Read the model definition and answer for the solid it produces. Units are mm, in the model's axes. Face numbers are marked on the shaded views. A direction names the side the tool comes from. Give positions to 0.01 mm unless a question says otherwise; leave off trailing zeros. Loops run counter-clockwise (first coordinate to the right, second up) from the corner with the lowest first, then second, coordinate; pieces in that order, holes last. Notation, with made-up numbers: (82.5, 30) - (131.5, 30) arc R26 cw to (131.5, 51) - close; hole circle Ø8 at (4, 87.5). An arc over 180 degrees is marked (long way). Write each question's results on one line, items separated by ' | '. Start each with the question number.
Q1. Find the intervals of material crossed by line 1 (Y direction, x = 5, z = -6); line 2 (Y direction, x = -2, z = -7.5); line 3 (Z direction, x = -7.5, y = -39), in increasing order. Write a range as from..to.
Q2. Determine the mould class of the marked faces 1, 2 and 3 for opening direction X: +X half, -X half, draft (parallel to the pull), parting line (faces both ways), or undercut.
Q3. Given pin 1 (10 mm diameter, centred on y = -39.5, z = -2.5, fed in from +X); pin 2 (12 mm diameter, centred on x = -7.5, z = 21.5, fed in from +Y); pin 3 (13.5 mm diameter, centred on x = -7, y = -42.5, fed in from -Z); pin 4 (7.5 mm diameter, centred on x = 2.86, y = 9.6, fed in from +Z), each flat-ended and moving along its own axis, determine where each tip first touches the part or whether it passes through.
Q4. The part is cut by section B-B, the plane y = -26.5. Write down the section's boundary in (x, z) (3 decimals), plus the area to 3 significant figures.
Q5. For the marked faces 4, 5 and 6, determine the directions among +Z, -Z, +X, -X, +Y, -Y from which every point of the face is accessible in a straight line to the end or side of a thin tool.
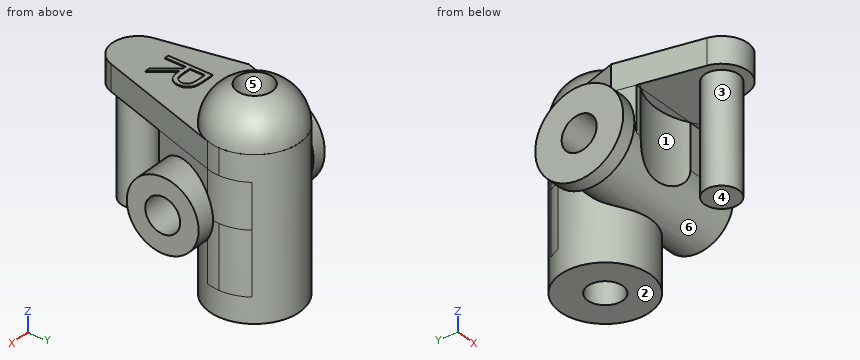
```python
from build123d import *
from build123d.topology import SkipClean

# Parameters (mm, degrees)
BOSS_EXTRU_1_DEPTH      = 1.45
ESQUISSE2_R             = 2.5
BOSS_EXTRU_2_DEPTH      = 2.2
BOSS_EXTRU_3_START      = -11.05
ESQUISSE3_R             = 2.5
BOSS_EXTRU_3_DEPTH      = 11.05
BOSS_EXTRU_4_START      = -1.45
ESQUISSE4_R             = 0.95
BOSS_EXTRU_4_DEPTH      = 7.5
CONG_1_R                = 2.2
BOSS_EXTRU_5_DEPTH      = 1
BOSS_EXTRU_5_DEPTH_BACK = 7.454
ENL_V_START             = -6
ENL_V_MAT_EXTRU_2_DEPTH = 6
BOSS_EXTRU_6_DEPTH      = 1
BOSS_EXTRU_6_DEPTH_BACK = 7.45
ESQUISSE8_R             = 2
ESQUISSE9_R             = 2.45
BOSS_EXTRU_7_DEPTH      = 0.8
ENL_V_START_2           = -6.05
ESQUISSE10_R            = 3.6
ESQUISSE10_R_2          = 0.95
ENL_V_MAT_EXTRU_3_DEPTH = 6.05
ESQUISSE11_R            = 0.975
ENL_V_MAT_EXTRU_4_DEPTH = 14.8
ESQUISSE12_R            = 0.975
ENL_V_MAT_EXTRU_5_DEPTH = 14.8
BOSS_EXTRU_8_DEPTH      = 0.05
SCALE1_SCALE            = 6.5


with BuildPart() as part:
    # Esquisse1 → Boss.-Extru.1 (new body)
    with BuildSketch(Plane.XY):
        with BuildLine():
            Line((2.388668556, -0.737741507), (0.152544962, -7.977890074))
            ThreePointArc((0.152544962, -7.977890074), (-1.300802178, -8.998408422), (-2.652272655, -7.846365386))
            Line((-2.652272655, -7.846365386), (-3.615331703, -3.23396357))
            Line((-3.615331703, -3.23396357), (-2.388668556, 0.737741507))
            ThreePointArc((-2.388668556, 0.737741507), (0.737741507, 2.388668556), (2.388668556, -0.737741507))
        make_face()
    extrude(amount=BOSS_EXTRU_1_DEPTH)

    # Esquisse2 → Boss.-Extru.2 (add)
    with BuildSketch(Plane.XY.offset(1.45)):
        with Locations(Location((0, 0, 0), (0, 0, 162.836669811))):
            Circle(ESQUISSE2_R)
    extrude(amount=BOSS_EXTRU_2_DEPTH)

    # Esquisse3 → Boss.-Extru.3 (add)
    with BuildSketch(Plane.XY.offset(3.65).offset(BOSS_EXTRU_3_START)):
        Circle(ESQUISSE3_R)
    extrude(amount=BOSS_EXTRU_3_DEPTH)

    # Esquisse4 → Boss.-Extru.4 (add)
    with BuildSketch(Plane(origin=(0, 0, 0), x_dir=(-1, 0, 0), z_dir=(0, 0, -1)).offset(BOSS_EXTRU_4_START)):
        with Locations(Location((1.232882801, -7.55, 0), (0, 0, 180))):
            Circle(ESQUISSE4_R)
    extrude(amount=BOSS_EXTRU_4_DEPTH)

    # Congé1
    cong_1_edges = [part.edges().sort_by_distance(p)[0] for p in [
        (2.388668556, -0.737741507, 3.65),
    ]]
    fillet(cong_1_edges, radius=CONG_1_R - 0.0001)  # a hair under: the kernel refuses the full size

    # Esquisse5 → Boss.-Extru.5 (add, two sides: drawn at the far end of the back side and taken through both)
    with SkipClean():  # the faces are left unmerged after this step: merging them gives an invalid solid
        with BuildSketch(Plane(origin=(2.499733458, 0.03650531, 0), x_dir=(0, 0, -1), z_dir=(0.9998933833040308, 0.014602123983129264, 0)).offset(-BOSS_EXTRU_5_DEPTH_BACK)):
            with BuildLine():
                Line((2.5, -4.4), (0, -4.4))
                Line((0, -4.4), (0, 1.44275903))
                Line((0, 1.44275903), (2.5, 1.44275903))
                Line((2.5, 1.44275903), (2.5, -0.4))
                ThreePointArc((2.5, -0.4), (4.5, -2.4), (2.5, -4.4))
            make_face()
        extrude(amount=BOSS_EXTRU_5_DEPTH + BOSS_EXTRU_5_DEPTH_BACK)
    add(part.part.scale(1), mode=Mode.REPLACE)  # the faces are merged on a copy

    # Esquisse7 → Enlèv. mat.-Extru.2 (cut)
    with SkipClean():  # the faces are left unmerged after this step: merging them gives an invalid solid
        with BuildSketch(Plane.XY.offset(ENL_V_START)):
            with BuildLine():
                Line((-2.062527014, 1.412792382), (-4.974539167, 1.370266286))
                Line((-4.974539167, 1.370266286), (-4.889222475, -4.471869809))
                Line((-4.889222475, -4.471869809), (-3.361517986, -4.4495597))
                Line((-3.361517986, -4.4495597), (-3.615331703, -3.23396357))
                Line((-3.615331703, -3.23396357), (-2.388668556, 0.737741507))
                ThreePointArc((-2.388668556, 0.737741507), (-2.251046184, 1.087561988), (-2.062527014, 1.412792382))
            make_face()
            with BuildLine():
                Line((1.263130408, -4.38202281), (3.563876187, -4.348423453))
                Line((3.563876187, -4.348423453), (3.478559495, 1.493712642))
                Line((3.478559495, 1.493712642), (2.020392322, 1.472418034))
                ThreePointArc((2.020392322, 1.472418034), (2.46599995, 0.410906614), (2.388668556, -0.737741507))
                Line((2.388668556, -0.737741507), (1.263130408, -4.38202281))
            make_face()
        extrude(amount=ENL_V_MAT_EXTRU_2_DEPTH, mode=Mode.SUBTRACT)
    add(part.part.scale(1), mode=Mode.REPLACE)  # the faces are merged on a copy

    # Esquisse8 → Boss.-Extru.6 (add, two sides: drawn at the far end of the back side and taken through both)
    with BuildSketch(Plane(origin=(2.499733458, 0.03650531, 0), x_dir=(0, 0, -1), z_dir=(0.9998933833040308, 0.014602123983129264, 0)).offset(-BOSS_EXTRU_6_DEPTH_BACK)):
        with Locations(Location((2.5, -2.4, 0), (0, 0, 90))):
            Circle(ESQUISSE8_R)
    extrude(amount=BOSS_EXTRU_6_DEPTH + BOSS_EXTRU_6_DEPTH_BACK)

    # Esquisse9 → Boss.-Extru.7 (add)
    with BuildSketch(Plane(origin=(-4.949472247, -0.072280514, 0), x_dir=(0, 0, 1), z_dir=(-0.9998933833040308, -0.014602123983129264, 0))):
        with Locations(Location((-2.5, -2.4, 0), (0, 0, 270))):
            Circle(ESQUISSE9_R)
    extrude(amount=-BOSS_EXTRU_7_DEPTH)

    # Esquisse10 → Enlèv. mat.-Extru.3 (cut)
    with BuildSketch(Plane(origin=(0, 0, -6.05), x_dir=(-1, 0, 0), z_dir=(0, 0, -1)).offset(ENL_V_START_2)):
        with Locations((1.232882801, -7.55)):
            Circle(ESQUISSE10_R)
        with Locations(Location((1.232882801, -7.55, 0), (0, 0, 180))):
            Circle(ESQUISSE10_R_2, mode=Mode.SUBTRACT)
    extrude(amount=ENL_V_MAT_EXTRU_3_DEPTH, mode=Mode.SUBTRACT)

    # Esquisse11 → Enlèv. mat.-Extru.4 (cut)
    with BuildSketch(Plane(origin=(0, 0, -7.4), x_dir=(-1, 0, 0), z_dir=(0, 0, -1))):
        Circle(ESQUISSE11_R)
    extrude(amount=-ENL_V_MAT_EXTRU_4_DEPTH, mode=Mode.SUBTRACT)

    # Esquisse12 → Enlèv. mat.-Extru.5 (cut)
    with BuildSketch(Plane(origin=(-4.949472247, -0.072280514, 0), x_dir=(0, 0, 1), z_dir=(-0.9998933833040308, -0.014602123983129264, 0))):
        with Locations(Location((-2.5, -2.4, 0), (0, 0, 270))):
            Circle(ESQUISSE12_R)
    extrude(amount=-ENL_V_MAT_EXTRU_5_DEPTH, mode=Mode.SUBTRACT)

    # Esquisse13 → Boss.-Extru.8 (add)
    with BuildSketch(Plane.XY.offset(1.45)):
        with BuildLine():
            Line((-1.885288931, -3.882291157), (-1.38498845, -3.882291157))
            add(Edge.make_bspline(
                [(-1.38498845, -3.882291157), (-1.35160193, -3.88240229), (-1.287496112, -3.882615677), (-1.195658062, -3.883805508), (-1.112210136, -3.887215762), (-1.037195965, -3.890150464), (-0.970616925, -3.895501851), (-0.912268861, -3.900616599), (-0.862420505, -3.907312071), (-0.832244897, -3.91353023), (-0.8185822, -3.916345644)],
                knots=[0, 0, 0, 0, 1.410062039, 2.707475311, 3.878576406, 4.937260626, 5.877586885, 6.699081471, 7.410979367, 8, 8, 8, 8], degree=3))
            add(Edge.make_bspline(
                [(-0.8185822, -3.916345644), (-0.800291754, -3.920864762), (-0.764101047, -3.929806594), (-0.711993857, -3.948706308), (-0.662340769, -3.970577469), (-0.615348037, -3.996265841), (-0.571251044, -4.025962112), (-0.529595107, -4.059153628), (-0.490191205, -4.095658775), (-0.454632898, -4.136397947), (-0.421105004, -4.179138311), (-0.392827413, -4.22535528), (-0.368451356, -4.273684943), (-0.349043844, -4.324618813), (-0.33341672, -4.377662936), (-0.322397978, -4.43329779), (-0.315789987, -4.491269915), (-0.315117233, -4.530811279), (-0.31477611, -4.550860869)],
                knots=[0, 0, 0, 0, 1.027469482, 2.033020251, 3.019912614, 3.986113645, 4.951240523, 5.91722682, 6.890402269, 7.87763091, 8.8651537, 9.85103654, 10.82876324, 11.815024772, 12.821070561, 13.842952187, 14.906261191, 16, 16, 16, 16], degree=3))
            add(Edge.make_bspline(
                [(-0.31477611, -4.550860869), (-0.315825395, -4.584171658), (-0.31787282, -4.649169635), (-0.33696218, -4.743498836), (-0.368231123, -4.831491203), (-0.411319186, -4.913035945), (-0.46619024, -4.986543548), (-0.53213652, -5.051108159), (-0.609194814, -5.105136668), (-0.680930039, -5.142602957), (-0.744297325, -5.166597892), (-0.796463977, -5.183481006), (-0.853368961, -5.196525267), (-0.914467057, -5.208211075), (-0.980012525, -5.217033714), (-1.049848267, -5.223495567), (-1.12402409, -5.227534173), (-1.174980568, -5.228135605), (-1.20119438, -5.228445003)],
                knots=[0, 0, 0, 0, 1.260483769, 2.459530307, 3.627416485, 4.787058657, 5.939039949, 7.08810263, 8.267026773, 9.491475466, 10.141966685, 10.831826277, 11.566392101, 12.351337768, 13.187381173, 14.07005841, 15.007169909, 16, 16, 16, 16], degree=3))
            Line((-1.20119438, -5.228445003), (-0.282724828, -6.382291157))
            Line((-0.282724828, -6.382291157), (-0.560168739, -6.382291157))
            Line((-0.560168739, -6.382291157), (-1.47863829, -5.228445003))
            Line((-1.47863829, -5.228445003), (-1.660929956, -5.228445003))
            Line((-1.660929956, -5.228445003), (-1.660929956, -6.382291157))
            Line((-1.660929956, -6.382291157), (-1.885288931, -6.382291157))
            Line((-1.885288931, -6.382291157), (-1.885288931, -3.882291157))
        make_face()
        with BuildLine():
            Line((-1.660929956, -4.138701413), (-1.660929956, -4.972034747))
            Line((-1.660929956, -4.972034747), (-1.203197585, -4.975540356))
            add(Edge.make_bspline(
                [(-1.203197585, -4.975540356), (-1.181826128, -4.975549811), (-1.140402159, -4.975568137), (-1.080473113, -4.972715439), (-1.024673033, -4.969470212), (-0.973215353, -4.964506394), (-0.926077085, -4.9581092), (-0.883281789, -4.950107068), (-0.84475961, -4.940784166), (-0.799832082, -4.926354433), (-0.749663131, -4.903492992), (-0.69514066, -4.870231921), (-0.648710419, -4.828396836), (-0.609483374, -4.780558653), (-0.577962352, -4.727961333), (-0.555739456, -4.671235355), (-0.541637711, -4.611812785), (-0.539974464, -4.570971279), (-0.539135085, -4.550360067)],
                knots=[0, 0, 0, 0, 1.146690395, 2.22261258, 3.21895312, 4.145990853, 4.996080663, 5.770904154, 6.481378293, 7.121626537, 8.300444488, 9.431385265, 10.535395872, 11.636531494, 12.74115979, 13.810798291, 14.895190096, 16, 16, 16, 16], degree=3))
            add(Edge.make_bspline(
                [(-0.539135085, -4.550360067), (-0.539993743, -4.530255372), (-0.541695289, -4.490415201), (-0.555587267, -4.432089551), (-0.579079682, -4.37704173), (-0.610738423, -4.325495669), (-0.649309248, -4.278705858), (-0.694536257, -4.238672177), (-0.745182825, -4.205636845), (-0.792519396, -4.184526573), (-0.834829547, -4.171583821), (-0.871565019, -4.162475847), (-0.913073217, -4.155158369), (-0.959555688, -4.149295468), (-1.010813995, -4.144256222), (-1.067107318, -4.140862095), (-1.128062161, -4.138852192), (-1.170309969, -4.138752843), (-1.192179956, -4.138701413)],
                knots=[0, 0, 0, 0, 1.101028733, 2.181837193, 3.264309656, 4.369019818, 5.486613113, 6.575447106, 7.666700264, 8.788928104, 9.402425223, 10.0903467, 10.862060571, 11.710948788, 12.657782767, 13.684531032, 14.801375019, 16, 16, 16, 16], degree=3))
            Line((-1.192179956, -4.138701413), (-1.660929956, -4.138701413))
        make_face(mode=Mode.SUBTRACT)
    extrude(amount=BOSS_EXTRU_8_DEPTH)


with BuildPart() as part_1:
    # Scale1: scaled about (-0.519885651, -1.745435598, -1.884204612)
    add(part.part.scale(SCALE1_SCALE).moved(Location((2.85937108, 9.599895789, 10.363125366))))


solid = part_1.part
```
Check sheet entries:
1) line 1: y = -18.39..-12.31, 0.37..3.63, 15.56..25.71 | line 2: y = -44.78..-34.17, -16.29..-12.2, 0.06..5.53, 13.67..25.11 | line 3: z = -28.96..19.79
2) face 1: undercut | face 2: draft | face 3: parting line
3) pin 1: stops at x = 1.02 | pin 2: stops at y = 25.21 | pin 3: stops at z = -28.96 | pin 4: passes through
4) outline: (-17.492, 10.363) - (8.717, 10.363) - (8.717, 19.788) - (-3.265, 19.788) - (-3.265, 20.113) - (-5.068, 20.113) - (-5.068, 19.788) - (-7.937, 19.788) - (-7.937, 20.113) - (-9.395, 20.113) - (-9.395, 19.788) - (-17.492, 19.788) - close | area: 248 mm^2
5) face 4: -Z, +X, -X, -Y | face 5: +Z, -Z | face 6: none
